Could you check a few things on this drawing? It's one solid part, dimensions in mm from its lowest x, y, z. Coordinates: 2 decimals unless noted, no trailing zeros. Write each loop counter-clockwise with the first axis right and the second up, starting at its lowest first coordinate (ties: lowest second). Pieces come first, ordered by that corner, then holes.
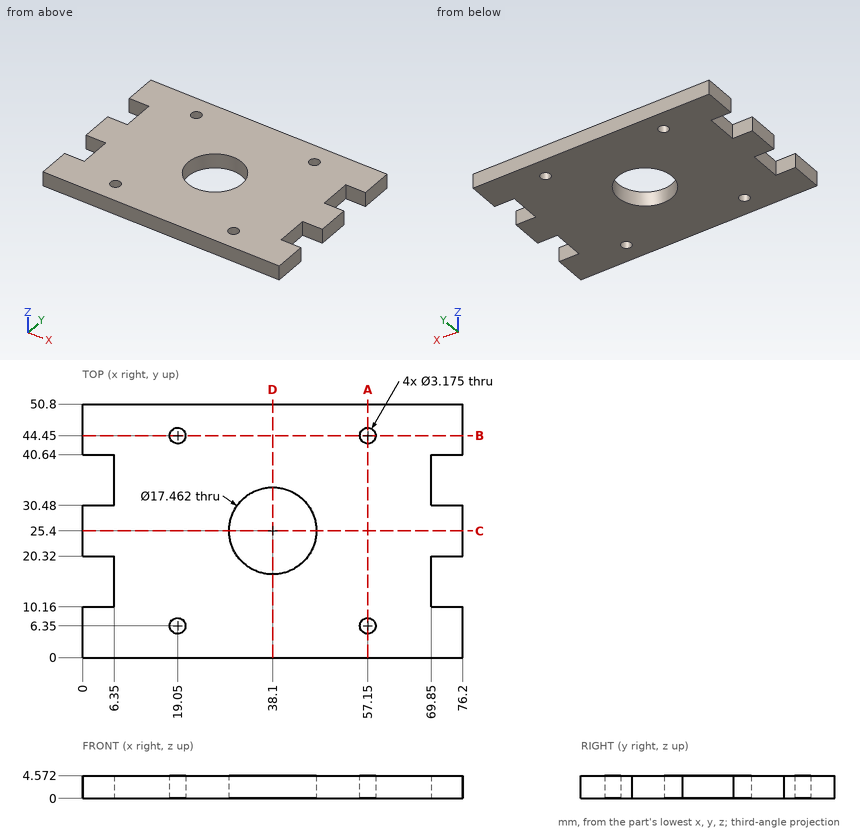
1) Will these pins go through, and if not, where does the flat tip stop? pin 1 (2.5 mm diameter, centred on y = 15, z = 3.5, fed in from -X); pin 2 (4 mm diameter, centred on x = 19.05, y = 6.35, fed in from +Z); pin 3 (2 mm diameter, centred on y = 32.5, z = 4, fed in from +X); pin 4 (1.9 mm diameter, centred on x = 19.05, y = 44.45, fed in from +Z).
Values follow:
pin 1: stops at x = 6.35
pin 2: stops at z = 4.57
pin 3: stops at x = 69.85
pin 4: passes through
2) Imagine slicing it at D-D on x = 38.1. Please give me the cut outline in (y, z).
Values follow:
outline: (0, 0) - (16.67, 0) - (16.67, 4.57) - (0, 4.57) - close; (34.13, 0) - (50.8, 0) - (50.8, 4.57) - (34.13, 4.57) - close
3) Imagine slicing it at C-C on y = 25.4. Please give me the cut outline in (x, z).
Values follow:
outline: (0, 0) - (29.37, 0) - (29.37, 4.57) - (0, 4.57) - close; (46.83, 0) - (76.2, 0) - (76.2, 4.57) - (46.83, 4.57) - close
4) I need wall thicknesses on probe 1 along Y at (x, z) = (4, 1.25); probe 2 along Y at (x, z) = (19.05, 2.15); probe 3 along Y at (x, z) = (38.1, 2.55). Which ranges of each line are inside material? Lowest first, please.
Values follow:
probe 1: y = 0 to 10.16, 20.32 to 30.48, 40.64 to 50.8
probe 2: y = 0 to 4.76, 7.94 to 42.86, 46.04 to 50.8
probe 3: y = 0 to 16.67, 34.13 to 50.8
5) Imagine slicing it at A-A on x = 57.15. Please give me the cut outline in (y, z).
Values follow:
outline: (0, 0) - (4.76, 0) - (4.76, 4.57) - (0, 4.57) - close; (7.94, 0) - (42.86, 0) - (42.86, 4.57) - (7.94, 4.57) - close; (46.04, 0) - (50.8, 0) - (50.8, 4.57) - (46.04, 4.57) - close
6) Imagine slicing it at B-B on y = 44.45. Please give me the cut outline in (x, z).
Values follow:
outline: (0, 0) - (17.46, 0) - (17.46, 4.57) - (0, 4.57) - close; (20.64, 0) - (55.56, 0) - (55.56, 4.57) - (20.64, 4.57) - close; (58.74, 0) - (76.2, 0) - (76.2, 4.57) - (58.74, 4.57) - close
